Geometry check sheet. Reference: drawing and pictorial views, mm from the part's lowest x, y, z. A direction names the side the tool comes from. Give positions to 0.01 mm unless a question says otherwise; leave off trailing zeros. Order: outer loops, then holes, each group sorted by start corner. A loop starts at its lowest first (then second) coordinate and runs counter-clockwise, first axis right, second up. Notation, with made-up numbers: (57.5, -16) -> (62.5, -16) arc R30 cw to (62.5, 23) -> close; hole circle Ø10 at (17.5, 5.5). An arc over 180 degrees is marked (long way). Write each question's results on one line, items separated by ' | '.
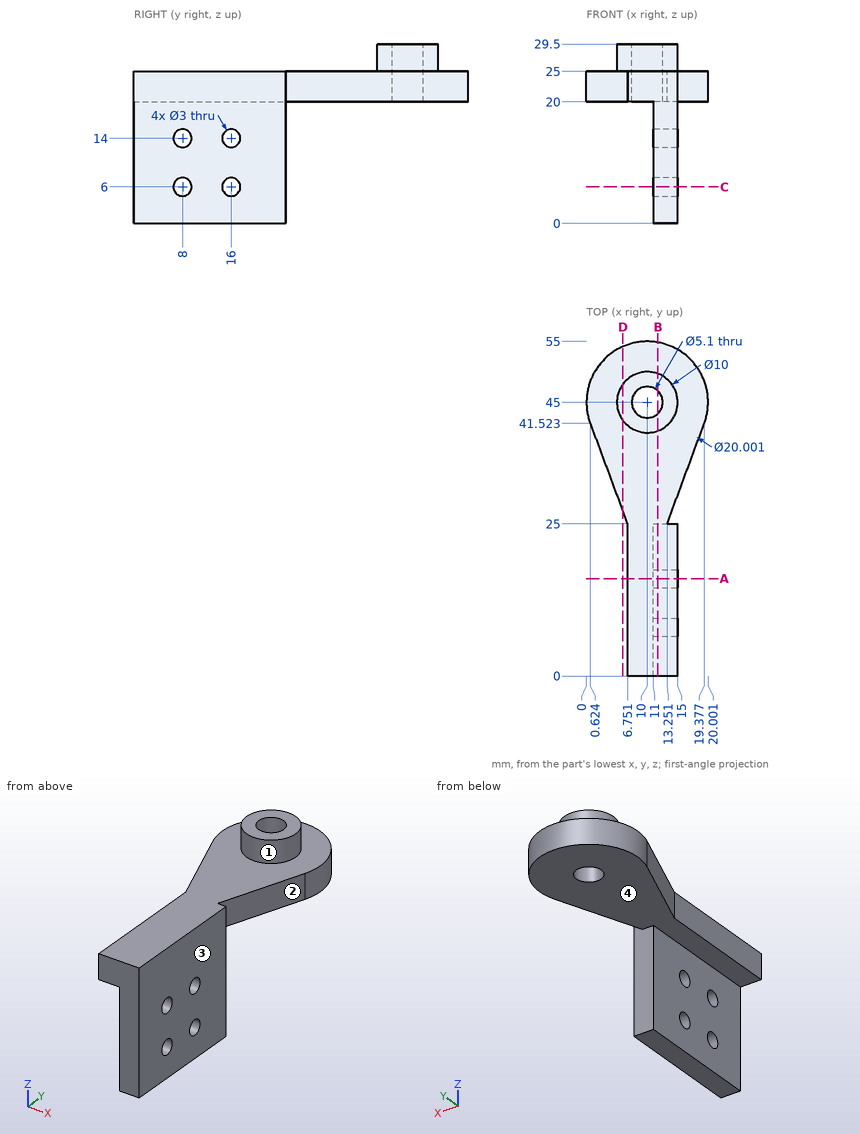
1. Section check D-D on x = 6. Record the cut outline in (y, z) (1 decimal).
Verdict:
outline: (27, 20) -> (54.2, 20) -> (54.2, 25) -> (48, 25) -> (48, 29.5) -> (42, 29.5) -> (42, 25) -> (27, 25) -> close
2. Section check A-A on y = 16. Record the cut outline in (x, z).
Verdict:
outline: (6.75, 20) -> (11, 20) -> (11, 15.5) -> (15, 15.5) -> (15, 25) -> (6.75, 25) -> close; (11, 0) -> (15, 0) -> (15, 4.5) -> (11, 4.5) -> close; (11, 7.5) -> (15, 7.5) -> (15, 12.5) -> (11, 12.5) -> close
3. Section check C-C on z = 6. Record the cut outline in (x, y).
Verdict:
outline: (11, 0) -> (15, 0) -> (15, 6.5) -> (11, 6.5) -> close; (11, 9.5) -> (15, 9.5) -> (15, 14.5) -> (11, 14.5) -> close; (11, 17.5) -> (15, 17.5) -> (15, 25) -> (11, 25) -> close
4. Access from +Z, -Z, +X, -X, +Y, -Y to the whole of each face (thin tool, end or side, straight path). Record for the marked faces 1, 2, 3 and 4.
Verdict:
face 1: +Z | face 2: +Z, -Z, +X | face 3: +Z, -Z, +X, -Y | face 4: -Z, -X, +Y
5. Gauge pin test, flat ends, axial feed: pin 1 Ø16 at (y, z) = (17.5, 13) entering from -X; pin 2 Ø12 at (y, z) = (29.5, 10) entering from -X; pin 3 Ø4.5 at (x, z) = (12.5, 18) entering from +Y; pin 4 Ø2.5 at (y, z) = (8, 6) entering from -X. Record the tip position at first contact, or that the pin passes through.
Verdict:
pin 1: stops at x = 6.75 | pin 2: stops at x = 11 | pin 3: stops at y = 54.89 | pin 4: passes through
6. Material ranges on probe 1 along Y at (x, z) = (13.1, 6); probe 2 along Z at (x, y) = (12, 16); probe 3 along Y at (x, z) = (10.25, 23), recorded low to high. Write a range as from..to.
Verdict:
probe 1: y = 0..6.5, 9.5..14.5, 17.5..25 | probe 2: z = 0..4.5, 7.5..12.5, 15.5..25 | probe 3: y = 0..42.46, 47.54..55
7. Section check B-B on x = 11.75. Record the cut outline in (y, z) (1 decimal), then the cut area to 3 significant figures.
Verdict:
outline: (0, 0) -> (25, 0) -> (25, 20) -> (43.1, 20) -> (43.1, 29.5) -> (40.3, 29.5) -> (40.3, 25) -> (0, 25) -> close; (46.9, 20) -> (54.8, 20) -> (54.8, 25) -> (49.7, 25) -> (49.7, 29.5) -> (46.9, 29.5) -> close; hole circle Ø3 at (8, 6); hole circle Ø3 at (8, 14); hole circle Ø3 at (16, 6); hole circle Ø3 at (16, 14) | area: 753 mm^2
